Input: dimensioned drawing with shaded views. Units: mm. Origin: part minimum x, y, z. A direction names the side the tool comes from. Round coordinates to 2 decimals unless told otherwise and drop trailing zeros. Order: outer loops, then holes, each group sorted by start corner. A loop starts at its lowest first (then second) coordinate and runs counter-clockwise, first axis right, second up. Notation, with made-up numbers: (61, 38) - (101, 38) arc R22 ccw to (101, 53) - close; hole circle Ø2 at (-19.5, 14.5). An arc over 180 degrees is marked (long way). Return JSON: item names as keys, results as strings. Group by question number.
1) Access query for the marked faces 1, 2, 3, 4 and 5. Directions: +Z, -Z, +X, -X, +Y, -Y. A direction counts if a zero-diameter tool reaches every point of the face in a straight line with its end or side. Return the directions, or none.
2) Section C-C, the plane z = 13.5. Return loops of the section in (x, y).
3) Contact query for flat-ended pins moving along their axis: P1, Ø1.5, axis at x = 44.5, y = 12, coming from the -Z side; P2, Ø5.5, axis at x = 5, y = 12, coming from the -Z side; P3, Ø11, axis at x = 3.5, z = 20, coming from the +Y side; P4, Ø2.5, axis at y = 10.5, z = 3.5, coming from the -X side. Output: stop coordinate, or through.
4) Section B-B, the plane z = 30.5. Return loops of the section in (x, y), plus the area to 3 significant figures.
5) Ray query, line 1 (X direction, y = 12, z = 29.15); line 2 (X direction, y = 1, z = 12); line 3 (Y direction, x = 48, z = 30). Return the intervals inside material, ascending. Write a range as from..to.
6) Mould query, pull axis Y, two halves, no side actions, for the marked faces 6, 7 and 8. Classes: pulls with the +Y half, pulls with the -Y half, needs draft (parallel to the pull), parting line crosses it, or undercut.
7) Section A-A, the plane x = 48. Return loops of the section in (y, z), plus the area to 3 significant figures.
8) Section D-D, the plane x = 34. Return loops of the section in (y, z).
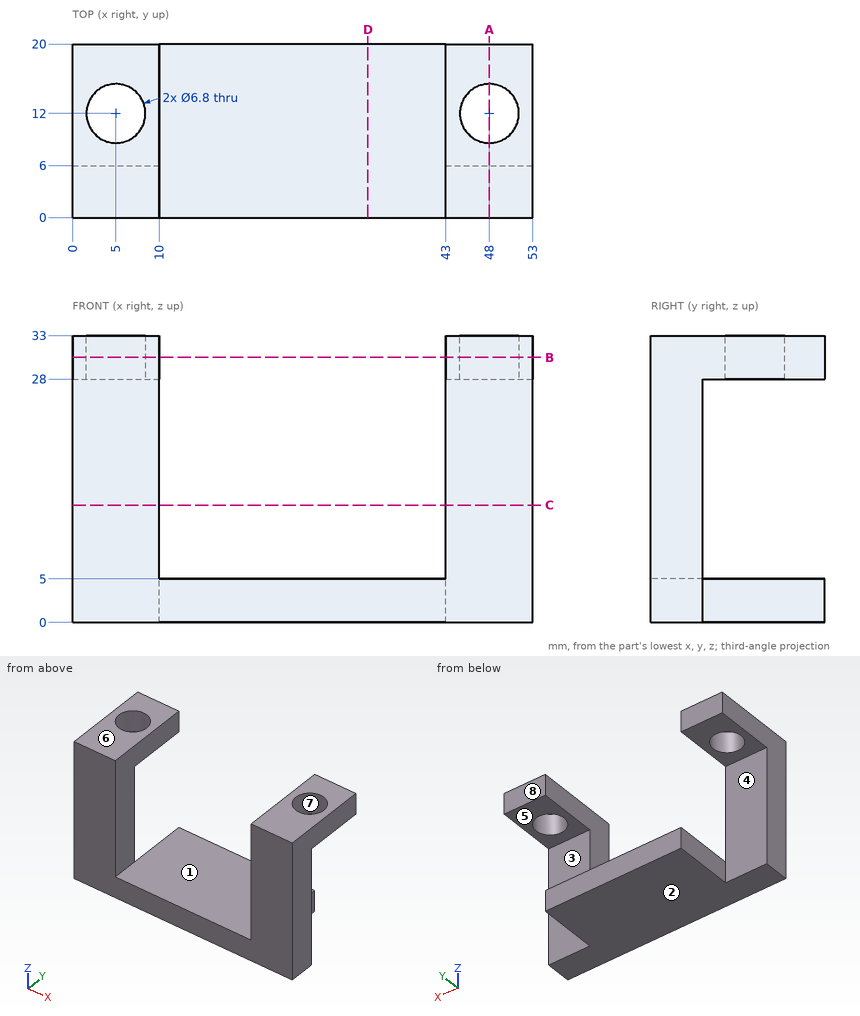
Geometry check:
{
 "1": {"face 1": "+Z, +Y, -Y", "face 2": "-Z, +X, -X, +Y, -Y", "face 3": "-Z, +X, +Y", "face 4": "-Z, -X, +Y", "face 5": "-Z, +X, -X, +Y"},
 "2": {"outline": "(0, 0) - (10, 0) - (10, 6) - (0, 6) - close; (43, 0) - (53, 0) - (53, 6) - (43, 6) - close"},
 "3": {"P1": "z = 28", "P2": "through", "P3": "y = 6", "P4": "x = 10"},
 "4": {"outline": "(0, 0) - (10, 0) - (10, 20) - (0, 20) - close; (43, 0) - (53, 0) - (53, 20) - (43, 20) - close; hole circle Ø6.8 at (5, 12); hole circle Ø6.8 at (48, 12)", "area": "327 mm2"},
 "5": {"line 1": "0..1.6, 8.4..10, 43..44.6, 51.4..53", "line 2": "0..10, 43..53", "line 3": "0..8.6, 15.4..20"},
 "6": {"face 6": "needs draft", "face 7": "undercut", "face 8": "pulls with the +Y half"},
 "7": {"outline": "(0, 0) - (6, 0) - (6, 28) - (8.6, 28) - (8.6, 33) - (0, 33) - close; (15.4, 28) - (20, 28) - (20, 33) - (15.4, 33) - close", "area": "234 mm2"},
 "8": {"outline": "(0, 0) - (20, 0) - (20, 5) - (0, 5) - close"}
}
